```python
from build123d import *

# Parameters (mm, degrees)
F1_DEPTH = 22.3
F3_D     = 11.5
F4_DEPTH = 5
F5_DEPTH = 22.3


with BuildPart() as f1:
    # F0 (on Front) → F1 (new body, symmetric)
    with BuildSketch(Plane.XZ):
        Polygon((59.7, 25.25), (38.1, 25.25), (-38.1, 25.25), (-38.1, 20.25), (38.1, 20.25), (59.7, 20.25), align=None)
    extrude(amount=F1_DEPTH, both=True)

    # F3 (through all)
    with Locations(Plane.XY.offset(25.25)):
        with Locations((-21.6, 11.25), (0, 11.25), (21.6, 11.25), (21.6, -11.25), (0, -11.25), (-21.6, -11.25), (43.2, 11.25), (43.2, -11.25)):
            Hole(F3_D / 2)

    # F0 (on Front) → F4 (join, symmetric)
    with BuildSketch(Plane.XZ):
        with BuildLine():
            Line((38.1, 20.25), (-38.1, 20.25))
            Line((-38.1, 20.25), (-38.1, -2.75))
            Line((-38.1, -2.75), (-27.8, -2.75))
            ThreePointArc((-27.8, -2.75), (-21.6, 3.45), (-15.4, -2.75))
            Line((-15.4, -2.75), (-6.2, -2.75))
            ThreePointArc((-6.2, -2.75), (0, 3.45), (6.2, -2.75))
            Line((6.2, -2.75), (15.4, -2.75))
            ThreePointArc((15.4, -2.75), (21.6, 3.45), (27.8, -2.75))
            Line((27.8, -2.75), (37, -2.75))
            ThreePointArc((37, -2.75), (43.2, 3.45), (49.4, -2.75))
            Line((49.4, -2.75), (59.7, -2.75))
            Line((59.7, -2.75), (59.7, 20.25))
            Line((59.7, 20.25), (38.1, 20.25))
        make_face()
        with BuildLine():
            Line((-27.8, -2.75), (-38.1, -2.75))
            Line((-38.1, -2.75), (-38.1, -20.25))
            Line((-38.1, -20.25), (38.1, -20.25))
            Line((38.1, -20.25), (59.7, -20.25))
            Line((59.7, -20.25), (59.7, -2.75))
            Line((59.7, -2.75), (49.4, -2.75))
            ThreePointArc((49.4, -2.75), (43.2, -8.95), (37, -2.75))
            Line((37, -2.75), (27.8, -2.75))
            ThreePointArc((27.8, -2.75), (21.6, -8.95), (15.4, -2.75))
            Line((15.4, -2.75), (6.2, -2.75))
            ThreePointArc((6.2, -2.75), (0, -8.95), (-6.2, -2.75))
            Line((-6.2, -2.75), (-15.4, -2.75))
            ThreePointArc((-15.4, -2.75), (-21.6, -8.95), (-27.8, -2.75))
        make_face()
    extrude(amount=F4_DEPTH, both=True)

    # F0 (on Front) → F5 (join, symmetric)
    with BuildSketch(Plane.XZ):
        Polygon((38.1, -20.25), (-38.1, -20.25), (-38.1, -25.25), (38.1, -25.25), (59.7, -25.25), (59.7, -20.25), align=None)
    extrude(amount=F5_DEPTH, both=True)


solid = f1.part
```
Work out the finished part from the listing and answer in its coordinate system (mm). A direction names the side the tool comes from. Give positions to 0.01 mm unless a question says otherwise; leave off trailing zeros. Loops run counter-clockwise (first coordinate to the right, second up) from the corner with the lowest first, then second, coordinate; pieces in that order, holes last. Notation, with made-up numbers: (22, 15.5) -> (59, 15.5) arc R20 cw to (59, 29.5) -> close; hole circle Ø11 at (-37, 84.5). An arc over 180 degrees is marked (long way). Write item = value, one per line. Start each with the question number.
(1) The mould has two halves that part along Y. Classify faces 1 (the flat face through (10, 22.3, -23)), 2 (the cylindrical face through (-27.084, 12.977, 22.715)), 3 (the flat face through (-38.1, 0, 0)): +Y half, -Y half, draft (parallel to the pull), parting line (faces both ways), or undercut.
(2) Find the intervals of material crossed by probe 1 along X at (y, z) = (11, 21); probe 2 along Z at (x, y) = (38.5, 18); probe 3 along X at (y, z) = (12.5, 20.5), in increasing order. Write a range as from..to.
(3) Find section B-B on x = -21.6. Give the vertices of the cut face in (y, z), and give its area (3 significant figures).
(4) Which of the six approach directions +Z, -Z, +X, -X, +Y, -Y give full straight-line access (tool end or side, diameter ignored) to faces 4 (the cylindrical face through (0.75, -5.55, 22.72)), 5 (the flat face through (11, -14, -20.25)), 6 (the cylindrical face through (38.28, -0.07, 1.02)), 7 (the flat face through (11, 14, -20.25))?
(5) Given pin 1 Ø7 at (x, y) = (43.2, -11.25) entering from +Z; pin 2 Ø3 at (x, z) = (-2, 7.5) entering from +Y; pin 3 Ø20 at (x, z) = (0, -2.75) entering from -Y; pin 4 Ø10 at (x, z) = (-21.6, -2.75) entering from -Y, each flat-ended and moving along its own axis, determine where each tip first touches the part or whether it passes through.
(6) Find section D-D on y = 19.5. Give the vertices of the cut face in (x, z), and give its area (3 significant figures).
(7) Find section A-A on y = -11.25. Give the vertices of the cut face in (x, z), and give its area (3 significant figures).
(8) Find section C-C on z = -2.75. Give the vertices of the cut face in (x, y), and give its area (3 significant figures).
From the geometry:
q1.face_1 = +Y half
q1.face_2 = undercut
q1.face_3 = draft
q2.probe_1 = -38.1..-27.34, -15.86..-5.74, 5.74..15.86, 27.34..37.46, 48.94..59.7
q2.probe_2 = -25.25..-20.25, 20.25..25.25
q2.probe_3 = -38.1..-27.21, -15.99..-5.61, 5.61..15.99, 27.21..37.59, 48.81..59.7
q3.outline = (-22.3, -25.25) -> (22.3, -25.25) -> (22.3, -20.25) -> (5, -20.25) -> (5, -8.95) -> (-5, -8.95) -> (-5, -20.25) -> (-22.3, -20.25) -> close; (-22.3, 20.25) -> (-17, 20.25) -> (-17, 25.25) -> (-22.3, 25.25) -> close; (-5.5, 20.25) -> (-5, 20.25) -> (-5, 3.45) -> (5, 3.45) -> (5, 20.25) -> (5.5, 20.25) -> (5.5, 25.25) -> (-5.5, 25.25) -> close; (17, 20.25) -> (22.3, 20.25) -> (22.3, 25.25) -> (17, 25.25) -> close
q3.area = 612 mm^2
q4.face_4 = +Z
q4.face_5 = +X, -X, -Y
q4.face_6 = +Y, -Y
q4.face_7 = +X, -X, +Y
q5.pin_1 = -20.25
q5.pin_2 = 5
q5.pin_3 = -5
q5.pin_4 = through
q6.outline = (-38.1, -25.25) -> (59.7, -25.25) -> (59.7, -20.25) -> (-38.1, -20.25) -> close; (-38.1, 20.25) -> (59.7, 20.25) -> (59.7, 25.25) -> (-38.1, 25.25) -> close
q6.area = 978 mm^2
q7.outline = (-38.1, -25.25) -> (59.7, -25.25) -> (59.7, -20.25) -> (-38.1, -20.25) -> close; (-38.1, 20.25) -> (-27.35, 20.25) -> (-27.35, 25.25) -> (-38.1, 25.25) -> close; (-15.85, 20.25) -> (-5.75, 20.25) -> (-5.75, 25.25) -> (-15.85, 25.25) -> close; (5.75, 20.25) -> (15.85, 20.25) -> (15.85, 25.25) -> (5.75, 25.25) -> close; (27.35, 20.25) -> (37.45, 20.25) -> (37.45, 25.25) -> (27.35, 25.25) -> close; (48.95, 20.25) -> (59.7, 20.25) -> (59.7, 25.25) -> (48.95, 25.25) -> close
q7.area = 748 mm^2
q8.outline = (-38.1, -5) -> (-27.8, -5) -> (-27.8, 5) -> (-38.1, 5) -> close; (-15.4, -5) -> (-6.2, -5) -> (-6.2, 5) -> (-15.4, 5) -> close; (6.2, -5) -> (15.4, -5) -> (15.4, 5) -> (6.2, 5) -> close; (27.8, -5) -> (37, -5) -> (37, 5) -> (27.8, 5) -> close; (49.4, -5) -> (59.7, -5) -> (59.7, 5) -> (49.4, 5) -> close
q8.area = 482 mm^2
